Verification items for the finished model (mm, model axes). A direction names the side the tool comes from. Coordinates: 2 decimals unless noted, no trailing zeros. Order: outer loops, then holes, each group sorted by start corner. A loop starts at its lowest first (then second) coordinate and runs counter-clockwise, first axis right, second up. Notation, with made-up numbers: (-20.75, 3) -> (-8.75, 3) arc R6 cw to (-8.75, 12) -> close; hole circle Ø6 at (-1, -11). An arc over 180 degrees is marked (long way). Answer as CSV lines item,"result".
Autodesk Inventor part; units mm, degrees
ref_plane "YZ Plane" through (0, 0, 0) normal (1, 0, 0) x (0, 1, 0)
ref_plane "XZ Plane" through (0, 0, 0) normal (0, 1, 0) x (-1, 0, 0)
ref_plane "XY Plane" through (0, 0, 0) normal (0, 0, 1) x (1, 0, 0)
sketch "Sketch1" plane through (0, 0, 0) normal (0, 1, 0) x (-1, 0, 0)
  line L0 (-17.5, -29.75) -> (17.5, -29.75)
  line L1 (17.5, -29.75) -> (17.5, 29.75)
  line L2 (17.5, 29.75) -> (-17.5, 29.75)
  line L3 (-17.5, 29.75) -> (-17.5, -29.75)
  line L4 (-17.5, -29.75) -> (17.5, 29.75) construction
  line L5 (17.5, -29.75) -> (-17.5, 29.75) construction
  point P0 (0, 0)
  dimension "d0" = 59.5
  dimension "d1" = 35
extrude "Extrusion1" add sketch "Sketch1" along normal blind 5
sketch "Sketch2" plane through (0, 5, 0) normal (0, 1, 0) x (1, 0, 0)
  line L0 (-17.5, -29.75) -> (17.5, -29.75)
  line L1 (15.25, -29.75) -> (-15.25, -29.75)
  line L2 (-15.25, -29.75) -> (-15.25, 27.5)
  line L3 (-15.25, 27.5) -> (15.25, 27.5)
  line L4 (15.25, 27.5) -> (15.25, -29.75)
  line L5 (17.5, -29.75) -> (17.5, 29.75)
  line L6 (17.5, 29.75) -> (-17.5, 29.75)
  line L7 (-17.5, 29.75) -> (-17.5, -29.75)
  point P0 (0, 0)
  point P1 (-15.25, -29.75)
  dimension "d4" = 2.25
  dimension "d5" = 2.25
  dimension "d6" = 2.25
extrude "Extrusion2" cut sketch "Sketch2" against normal blind 3 contours L2 L3 L4 L0
sketch "Sketch3" plane through (0, 2, 0) normal (0, 1, 0) x (1, 0, 0)
  line L0 (10.25, 15.5) -> (7.25, 15.5)
  line L1 (7.25, 15.5) -> (7.25, 12.5)
  line L2 (7.25, 12.5) -> (10.25, 12.5)
  line L3 (10.25, 12.5) -> (10.25, 15.5)
  line L4 (-15.25, 27.5) -> (15.25, 27.5)
  line L5 (15.25, 27.5) -> (15.25, -29.75)
  line L6 (15.25, -25.75) -> (12.75, -25.75)
  line L7 (12.75, -25.75) -> (12.75, -21.75)
  line L8 (12.75, -21.75) -> (15.25, -21.75)
  line L9 (15.25, -21.75) -> (15.25, -25.75)
  line L10 (-15.25, -29.75) -> (-15.25, 27.5)
  line L11 (-15.25, 11.5) -> (-12.75, 11.5)
  line L12 (-12.75, 11.5) -> (-12.75, 15.5)
  line L13 (-12.75, 15.5) -> (-15.25, 15.5)
  line L14 (-15.25, 15.5) -> (-15.25, 11.5)
  line L15 (15.25, -29.75) -> (-15.25, -29.75)
  point P0 (0, 0)
  point P1 (15.25, -21.75)
  dimension "d9" = 3
  dimension "d10" = 3
  dimension "d21" = 12
  dimension "d22" = 5
  dimension "d23" = 2.5
  dimension "d24" = 4
  dimension "d25" = 4
  dimension "d26" = 2.5
  dimension "d27" = 12
  dimension "d28" = 4
extrude "Extrusion3" add sketch "Sketch3" along normal blind 2 contours L3 L2 L1 L0
extrude "Extrusion4" add sketch "Sketch3" along normal blind 2.5 contours L13 L12 L11 L10 | L5 L6 L7 L8
sketch "Sketch4" plane through (0, 2, 0) normal (0, 1, 0) x (1, 0, 0)
  line L0 (11.1804, 11.7081) -> (6.3882, 11.7081)
  line L1 (6.3882, 11.7081) -> (6.3882, -25.8012)
  line L2 (6.3882, -25.8012) -> (11.1804, -25.8012)
  line L3 (11.1804, -25.8012) -> (11.1804, 11.7081)
  point P0 (0, 0)
extrude "Extrusion5" cut sketch "Sketch4" against normal through all
equation "\"d5\" = d4"
equation "\"d6\" = d4"
equation "\"d25\" = d24"
equation "\"d26\" = d23"
properties part number "CROC Gluing Form V1"
Item 1: Thickness scan on line 1 (X direction, y = 3.8, z = 15); line 2 (X direction, y = 0.5, z = 0); line 3 (Z direction, x = 8.5, y = 1.35). Record the ranges inside material, lowest first.
Answer list:
line 1,"-17.5 to -15.25, 15.25 to 17.5"
line 2,"-17.5 to 6.39, 11.18 to 17.5"
line 3,"-29.75 to -11.71, 25.8 to 29.75"
Item 2: Release check for a two-part mould opening along Z. For faces 6 (the flat face through (6.388, 1, 7)), 7 (the flat face through (14, 4.5, 24)), 8 (the flat face through (-14, 3, -11.5)), 9 (the flat face through (15.25, 4, 1)) record: +Z half, -Z half, draft (parallel to the pull), parting line (faces both ways), or undercut.
Answer list:
face 6,"undercut"
face 7,"draft"
face 8,"+Z half"
face 9,"undercut"
Item 3: Tool access check on faces 1 (the flat face through (0, 0, 0)), 2 (the flat face through (0, 2, -29.75)), 3 (the flat face through (11.18, 1, 7)), 4 (the flat face through (12.75, 3, 24)), 5 (the flat face through (-14, 3, -15.5)). Record the directions out of +Z, -Z, +X, -X, +Y, -Y that give a thin tool (end or side, any length) a straight path to the whole face; none if there is none.
Answer list:
face 1,"+Z, -Z, +X, -X, -Y"
face 2,"-Z, +X, -X, +Y, -Y"
face 3,"+Y, -Y"
face 4,"+Z, +Y"
face 5,"+Y"
Item 4: Depth check by flat-ended pin: pin 1 Ø3 at (x, y) = (14.5, 3) entering from +Z; pin 2 Ø3 at (x, z) = (5, -13.5) entering from +Y; pin 3 Ø0.8 at (x, y) = (-14, 3.5) entering from +Z; pin 4 Ø2.5 at (x, z) = (8, -14.5) entering from +Y. Enter the tip coordinate at first touch or a pass-through.
Answer list:
pin 1,"z = 29.75"
pin 2,"y = 2"
pin 3,"z = -11.5"
pin 4,"y = 4"
Item 5: Section check C-C, the plane x = -2. Record the boundary of the cut face in (y, z).
Answer list:
outline,"(0, -29.75) -> (5, -29.75) -> (5, -27.5) -> (2, -27.5) -> (2, 29.75) -> (0, 29.75) -> close"
Item 6: Section check A-A, the plane y = 2.65. Record the boundary of the cut face in (x, z).
Answer list:
outline,"(-17.5, -29.75) -> (17.5, -29.75) -> (17.5, 29.75) -> (15.25, 29.75) -> (15.25, 25.75) -> (12.75, 25.75) -> (12.75, 21.75) -> (15.25, 21.75) -> (15.25, -27.5) -> (-15.25, -27.5) -> (-15.25, -15.5) -> (-12.75, -15.5) -> (-12.75, -11.5) -> (-15.25, -11.5) -> (-15.25, 29.75) -> (-17.5, 29.75) -> close; (7.25, -15.5) -> (10.25, -15.5) -> (10.25, -12.5) -> (7.25, -12.5) -> close"
Item 7: Section check B-B, the plane z = 19. Record the boundary of the cut face in (x, y).
Answer list:
outline,"(-17.5, 0) -> (6.39, 0) -> (6.39, 2) -> (-15.25, 2) -> (-15.25, 5) -> (-17.5, 5) -> close; (11.18, 0) -> (17.5, 0) -> (17.5, 5) -> (15.25, 5) -> (15.25, 2) -> (11.18, 2) -> close"
Item 8: Section check D-D, the plane z = -17. Record the boundary of the cut face in (x, y), plus the area to 3 significant figures.
Answer list:
outline,"(-17.5, 0) -> (17.5, 0) -> (17.5, 5) -> (15.25, 5) -> (15.25, 2) -> (-15.25, 2) -> (-15.25, 5) -> (-17.5, 5) -> close"
area,"83.5 mm2"
